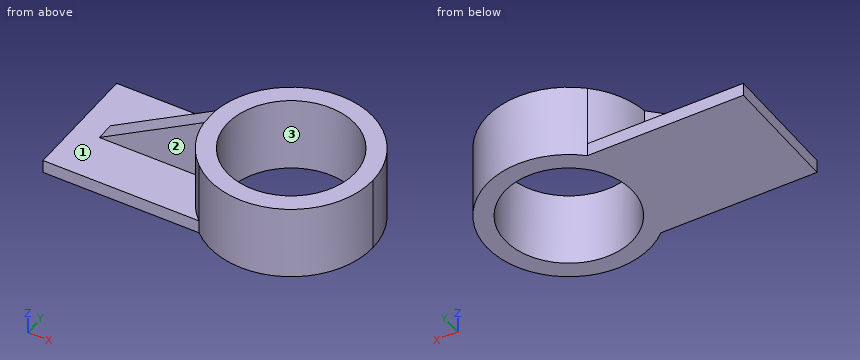
from build123d import *

# Parameters (mm, degrees)
F0_R     = 35.7057277328
F1_DEPTH = 41.656
F2_R     = 35.7057277328
F3_DEPTH = 34.29
F5_DEPTH = 25.4


with BuildPart() as f1:
    # F0 (on Top) → F1 (new body)
    with BuildSketch(Plane.XY):
        with BuildLine():
            Line((28.1166336854, 33.8129214942), (-58.9986741543, 33.8129214942))
            Line((-58.9986741543, 33.8129214942), (-58.9986741543, -33.8129214942))
            Line((-58.9986741543, -33.8129214942), (28.1166336854, -33.8129214942))
            ThreePointArc((28.1166336854, -33.8129214942), (13.2055078137, 0), (28.1166336854, 33.8129214942))
        make_face()
        with BuildLine():
            ThreePointArc((104.7918404949, 0), (77.4760612446, 41.8998836492), (28.1166336854, 33.8129214942))
            ThreePointArc((28.1166336854, 33.8129214942), (13.2055078137, 0), (28.1166336854, -33.8129214942))
            ThreePointArc((28.1166336854, -33.8129214942), (77.4760612446, -41.8998836492), (104.7918404949, 0))
        make_face()
        with Locations((58.9986741543, 0)):
            Circle(F0_R, mode=Mode.SUBTRACT)
    extrude(amount=F1_DEPTH)

    # F2 (on face) → F3 (cut)
    with BuildSketch(Plane.XY.offset(41.656)):
        with Locations((58.9986741543, 0)):
            Circle(F2_R)
        with BuildLine():
            ThreePointArc((13.4958462684, 5.1484694704), (18.2056020605, 20.8071947328), (28.1166336854, 33.8129214942))
            Line((28.1166336854, 33.8129214942), (-58.9986741543, 33.8129214942))
            Line((-58.9986741543, 33.8129214942), (-58.9986741543, -33.8129214942))
            Line((-58.9986741543, -33.8129214942), (28.1166336854, -33.8129214942))
            ThreePointArc((28.1166336854, -33.8129214942), (18.2056020605, -20.8071947328), (13.4958462684, -5.1484694704))
            Line((13.4958462684, -5.1484694704), (-45.0028181076, -5.1484694704))
            Line((-45.0028181076, -5.1484694704), (-45.0028181076, 5.1484694704))
            Line((-45.0028181076, 5.1484694704), (13.4958462684, 5.1484694704))
        make_face()
    extrude(amount=-F3_DEPTH, mode=Mode.SUBTRACT)

    # F4 (on face) → F5 (cut)
    with BuildSketch(Plane.XZ.offset(5.1484694704)):
        Polygon((-45.0028181076, 7.366), (13.4958462684, 41.656), (-45.0028181076, 41.656), align=None)
    extrude(amount=-F5_DEPTH, mode=Mode.SUBTRACT)


solid = f1.part
Work out the finished part from the listing and answer in its coordinate system (mm). Face numbers are marked on the shaded views. Give positions to 0.01 mm unless a question says otherwise; leave off trailing zeros. Write each loop counter-clockwise with the first axis right and the second up, starting at its lowest first coordinate (ties: lowest second). Pieces come first, ordered by that corner, then holes.
Q1. For a pull along Y with two mould halves and no side action, classify the marked faces 1, 2 and 3 as released by +Y, released by -Y, zero draft, split by the parting line, or undercut.
Answer:
face 1: zero draft
face 2: released by -Y
face 3: undercut
Q2. The part is cut by section B-B on x = 78.5. Give the vertices of the cut face in (y, z).
Answer:
outline: (-41.43, 0) - (-29.91, 0) - (-29.91, 41.66) - (-41.43, 41.66) - close; (29.91, 0) - (41.43, 0) - (41.43, 41.66) - (29.91, 41.66) - close
Q3. The part is cut by section C-C on y = 26. Give the vertices of the cut face in (x, z), and give its area (3 significant figures).
Answer:
outline: (-59, 0) - (34.53, 0) - (34.53, 41.66) - (21.3, 41.66) - (21.3, 7.37) - (-59, 7.37) - close; (83.47, 0) - (96.7, 0) - (96.7, 41.66) - (83.47, 41.66) - close
area: 1,690 mm2
Q4. Straight lines are drawn through the part: L1, parallel to Y at x = -37.5, z = 7.5; L2, parallel to X at y = -16, z = 33; L3, parallel to Z at x = -34.5, y = -12.5. For each, find the intervals that lie inside material, in ascending order.
Answer:
L1: y = -5.15 to 5.15
L2: x = 16.09 to 27.08, 90.92 to 101.91
L3: z = 0 to 7.37
Q5. The part is cut by section A-A on z = 4. Give the vertices of the cut face in (x, y).
Answer:
outline: (-59, -33.81) - (28.12, -33.81) arc R45.79 ccw (long way) to (28.12, 33.81) - (-59, 33.81) - close; hole circle Ø71.41 at (59, 0)
Q6. The part is cut by section D-D on x = -2.5. Give the vertices of the cut face in (y, z).
Answer:
outline: (-33.81, 0) - (33.81, 0) - (33.81, 7.37) - (5.15, 7.37) - (5.15, 32.28) - (-5.15, 32.28) - (-5.15, 7.37) - (-33.81, 7.37) - close
Q7. Given pin 1 (10 mm diameter, centred on x = 44, z = 15, fed in from +Y); pin 2 (8 mm diameter, centred on x = 3, z = 4.5, fed in from +Y); pin 3 (2 mm diameter, centred on x = 60, z = 7.5, fed in from +Y); pin 4 (17 mm diameter, centred on x = -5, z = 19, fed in from -Y), each flat-ended and moving along its own axis, determine where each tip first touches the part or whether it passes through.
Answer:
pin 1: stops at y = 44.69
pin 2: stops at y = 33.81
pin 3: stops at y = 45.79
pin 4: stops at y = -5.15
